Build history of the part. All positions in model axes, mm. Face numbers are marked on the shaded views. A direction names the side the tool comes from. Round coordinates to 2 decimals unless told otherwise and drop trailing zeros. Write each loop counter-clockwise with the first axis right and the second up, starting at its lowest first coordinate (ties: lowest second). Pieces come first, ordered by that corner, then holes. Notation, with made-up numbers: (89.25, -22.5) -> (148.25, -22.5) arc R30 ccw to (148.25, 14.5) -> close; hole circle Ø9 at (64, 5). An arc over 180 degrees is marked (long way). Return JSON: item names as keys, results as strings.
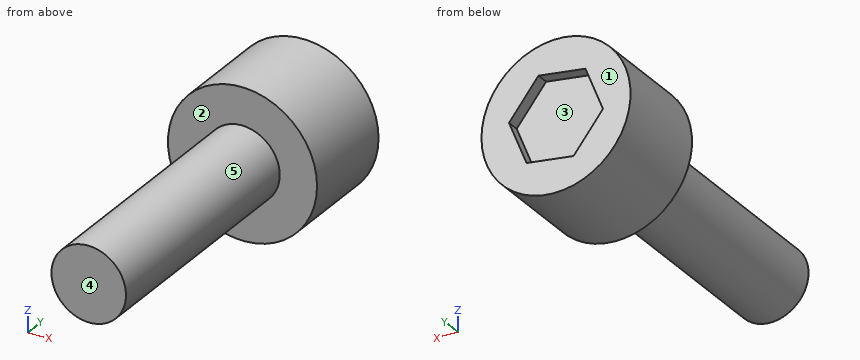
Autodesk Inventor part; units mm, degrees
ref_plane "YZ Plane" through (0, 0, 0) normal (1, 0, 0) x (0, 1, 0)
ref_plane "XZ Plane" through (0, 0, 0) normal (0, 1, 0) x (-1, 0, 0)
ref_plane "XY Plane" through (0, 0, 0) normal (0, 0, 1) x (1, 0, 0)
sketch "Sketch1" plane through (0, 0, 0) normal (0, 1, 0) x (-1, 0, 0)
  circle A0 centre (0, 0) radius 1.5
  dimension "d0" = 3
extrude "Extrusion1" add sketch "Sketch1" along normal blind 10
sketch "Sketch2" plane through (0, 10, 0) normal (0, 1, 0) x (1, 0, 0)
  circle A0 centre (0, 0) radius 3
  dimension "d3" = 6
extrude "Extrusion2" add sketch "Sketch2" along normal blind 4
sketch "Sketch3" plane through (0, 14, 0) normal (0, 1, 0) x (1, 0, 0)
  circle A0 centre (0, 0) radius 3
  line L0 (1.1834, 1.5) -> (1.8907, -0.2749)
  line L1 (1.8907, -0.2749) -> (0.7073, -1.7749)
  line L2 (0.7073, -1.7749) -> (-1.1834, -1.5)
  line L3 (-1.1834, -1.5) -> (-1.8907, 0.2749)
  line L4 (-1.8907, 0.2749) -> (-0.7073, 1.7749)
  line L5 (-0.7073, 1.7749) -> (1.1834, 1.5)
extrude "Extrusion3" cut sketch "Sketch3" against normal blind 0.5 contours L0 L1 L2 L3 L4 L5
thread "Thread1"
properties part number "M4 x10"
Q1. 3-axis set-ups, long thin cutter, end or side, ignore diameter. For the marked faces 1 and 2: which of +Z, -Z, +X, -X, +Y, -Y reach the whole face in a straight line?
Verdict:
{"face 1": "+Z, -Z, +X, -X, +Y", "face 2": "-Y"}
Q2. Saw through at B-B on x = 0.45. List the corners of the cut face in (y, z).
Verdict:
{"outline": "(0, -1.43) -> (10, -1.43) -> (10, -2.97) -> (14, -2.97) -> (14, -1.61) -> (13.5, -1.61) -> (13.5, 1.74) -> (14, 1.74) -> (14, 2.97) -> (10, 2.97) -> (10, 1.43) -> (0, 1.43) -> close"}
Q3. Saw through at A-A on z = -1.2. List the corners of the cut face in (x, y), then the cut area to 3 significant figures.
Verdict:
{"outline": "(-2.75, 10) -> (-0.9, 10) -> (-0.9, 0) -> (0.9, 0) -> (0.9, 10) -> (2.75, 10) -> (2.75, 14) -> (1.3, 14) -> (1.3, 13.5) -> (-1.16, 13.5) -> (-1.16, 14) -> (-2.75, 14) -> close", "area": "38.8 mm²"}
Q4. Saw through at D-D on x = -2.15. List the corners of the cut face in (y, z).
Verdict:
{"outline": "(10, -2.09) -> (14, -2.09) -> (14, 2.09) -> (10, 2.09) -> close"}
Q5. Pin check, flat tips, straight feed: pin 1 Ø2 at (x, y) = (-0.5, 8.5) entering from +Z; pin 2 Ø3 at (y, z) = (4, 1.5) entering from +X; pin 3 Ø1.8 at (x, z) = (0, 0) entering from +Y; pin 4 Ø1.5 at (x, z) = (0, -1.5) entering from -Y. Stop position of each tip, or through.
Verdict:
{"pin 1": "stops at z = 1.5", "pin 2": "stops at x = 1.5", "pin 3": "stops at y = 13.5", "pin 4": "stops at y = 0"}
Q6. Two-plate mould, pull along X, no slides. Class the marked faces 3, 4 and 5: +X half, -X half, draft (parallel to the pull), parting line (faces both ways), or undercut.
Verdict:
{"face 3": "undercut", "face 4": "draft", "face 5": "parting line"}
Q7. Saw through at C-C on y = 3. List the corners of the cut face in (x, z), then the cut area to 3 significant figures.
Verdict:
{"outline": "circle Ø3 at (0, 0)", "area": "7.07 mm²"}
Q8. Wall check: L1, parallel to Y at x = 0.15, z = 0.7; L2, parallel to Y at x = 0.9, z = 1.85; L3, parallel to Z at x = 0.1, y = 3.25. Give the ranges that are in metal, low to high.
Verdict:
{"L1": "y = 0 to 13.5", "L2": "y = 10 to 14", "L3": "z = -1.5 to 1.5"}
